Build history of the part. All positions in model axes, mm. A direction names the side the tool comes from. Round coordinates to 2 decimals unless told otherwise and drop trailing zeros. Order: outer loops, then holes, each group sorted by start corner. A loop starts at its lowest first (then second) coordinate and runs counter-clockwise, first axis right, second up. Notation, with made-up numbers: (-14.5, 19) - (34.5, 19) arc R10 cw to (34.5, 23) - close; hole circle Ø5 at (75, 76). An arc over 180 degrees is marked (long way). Write each question's results on one line, items separated by ' | '. Start each with the question number.
```python
from build123d import *

# Parameters (mm, degrees)
F0_R     = 25.4
F1_DEPTH = 88.9
F2_R     = 22.225
F3_DEPTH = 76.2
F4_R     = 21.59
F5_DEPTH = 12.7
F6_R     = 17.78
F7_DEPTH = 101.601


with BuildPart() as f1:
    # F0 (on Top) → F1 (new body)
    with BuildSketch(Plane.XY):
        Circle(F0_R)
    extrude(amount=F1_DEPTH)

    # F2 (on face) → F3 (cut)
    with BuildSketch(Plane.XY.offset(88.9)):
        Circle(F2_R)
    extrude(amount=-F3_DEPTH, mode=Mode.SUBTRACT)

    # F4 (on face) → F5 (join)
    with BuildSketch(Plane(origin=(0, 0, 0), x_dir=(1, 0, 0), z_dir=(0, 0, -1))):
        Circle(F4_R)
    extrude(amount=F5_DEPTH)

    # F6 (on face) → F7 (cut, through all)
    with BuildSketch(Plane(origin=(0, 0, -12.7), x_dir=(1, 0, 0), z_dir=(0, 0, -1))):
        Circle(F6_R)
    extrude(amount=-F7_DEPTH, mode=Mode.SUBTRACT)


solid = f1.part
```
1. Cut at C-C (z = 61). List the corners of the cut face in (x, y) (3 decimals).
2. 3-axis set-ups, long thin cutter, end or side, ignore diameter. For faces 4 (the face through (3, -18, -12.7)), 5 (the face through (-10, 15, 12.7)): which of +Z, -Z, +X, -X, +Y, -Y reach the whole face in a straight line?
3. Wall check: line 1 (Y direction, x = 0, z = 71.5) (3 decimals); line 2 (Y direction, x = 0, z = 0.25); line 3 (Z direction, x = 8.5, y = 16.5). Give the ranges that are in metal, low to high. Write a range as from..to.
4. Flat gauge pins, fed straight in: pin 1 Ø10 at (y, z) = (-17, 75) entering from -X; pin 2 Ø5 at (x, y) = (-1, 16.5) entering from -Z; pin 3 Ø4 at (x, z) = (-10.5, 48.5) entering from +Y; pin 4 Ø6 at (x, z) = (-15.5, 22.5) entering from -Y. Where does each tip first touch, or does it go through?
5. Mould opens along Y. For faces 1 (the face through (-3.85, 17.36, -0.18)), 2 (the face through (-11, -19, 0)), 3 (the face through (-15.913, -14.592, -6.261)) say: pulls with the +Y half, pulls with the -Y half, needs draft (parallel to the pull), parting line crosses it, or undercut.
6. Cut at A-A (x = 0). List the corners of the cut face in (y, z) (3 decimals).
A:
1) outline: circle Ø50.8 at (0, 0); hole circle Ø44.45 at (0, 0)
2) face 4: -Z, +X, -X, +Y, -Y | face 5: +Z
3) line 1: y = -25.4..-22.225, 22.225..25.4 | line 2: y = -25.4..-17.78, 17.78..25.4 | line 3: z = -12.7..12.7
4) pin 1: stops at x = -22.39 | pin 2: stops at z = -12.7 | pin 3: stops at y = 23.94 | pin 4: stops at y = -22.11
5) face 1: undercut | face 2: needs draft | face 3: parting line crosses it
6) outline: (-25.4, 0) - (-21.59, 0) - (-21.59, -12.7) - (-17.78, -12.7) - (-17.78, 12.7) - (-22.225, 12.7) - (-22.225, 88.9) - (-25.4, 88.9) - close; (17.78, -12.7) - (21.59, -12.7) - (21.59, 0) - (25.4, 0) - (25.4, 88.9) - (22.225, 88.9) - (22.225, 12.7) - (17.78, 12.7) - close
